```python
from build123d import *

# Parameters (mm, degrees)
F0_W     = 44.45
F0_H     = 38.1
F1_DEPTH = 19.05
F3_D     = 6.35
F3_DEPTH = 12.7
F3_TIP   = 1.9077324654
F5_D     = 6.35
F5_DEPTH = 12.7
F5_TIP   = 1.9077324654


with BuildPart() as f1:
    # F0 (on Right) → F1 (new body)
    with BuildSketch(Plane.YZ):
        with Locations((22.225, 19.05)):
            Rectangle(F0_W, F0_H)
    extrude(amount=F1_DEPTH)

    # F3
    with Locations(Plane.XY.offset(38.1)):
        with Locations((9.525, 22.225)):
            Hole(F3_D / 2, depth=F3_DEPTH)
            with Locations((0, 0, -(F3_DEPTH + F3_TIP / 2))):  # 118° drill point
                Cone(0, F3_D / 2, F3_TIP, mode=Mode.SUBTRACT)

    # F5
    with Locations(Plane(origin=(0, 0, 0), x_dir=(1, 0, 0), z_dir=(0, 0, -1))):
        with Locations((9.525, -12.7), (9.525, -31.75)):
            Hole(F5_D / 2, depth=F5_DEPTH)
            with Locations((0, 0, -(F5_DEPTH + F5_TIP / 2))):  # 118° drill point
                Cone(0, F5_D / 2, F5_TIP, mode=Mode.SUBTRACT)


solid = f1.part
```
Source: CAD feature listing. Evaluate the final solid. Frame: model axes, mm. A direction names the side the tool comes from. Give positions to 0.01 mm unless a question says otherwise; leave off trailing zeros. Loops run counter-clockwise (first coordinate to the right, second up) from the corner with the lowest first, then second, coordinate; pieces in that order, holes last. Notation, with made-up numbers: (-18, -36.75) - (14, -36.75) arc R20 ccw to (14, -11.75) - close; hole circle Ø2 at (-10.5, 71). An arc over 180 degrees is marked (long way). Use CSV: the item, a comma, the result in double quotes. Start each with the question number.
1. Ray query, L1, parallel to X at y = 12.7, z = 10; L2, parallel to Y at x = 7.75, z = 11.5; L3, parallel to X at y = 12, z = 7. Return the intervals inside material, ascending.
2. Section B-B (z = 29.5). Output: boundary loops of the cut face in (x, y) (3 decimals), then the cut area to 3 significant figures.
3. Section A-A (z = 3.5). Output: boundary loops of the cut face in (x, y) (3 decimals).
4. Reachability of faces 5 (the cylindrical face through (10.21, 34.85, 6.44)), 6 (the flat face through (0, 22, 19)), 7 (the cylindrical face through (9.938, 25.373, 31.661)) from +Z, -Z, +X, -X, +Y, -Y: full face, straight path, thin tool, end or side. Return the list, or none.
5. Pin query (flat end, axial travel): pin 1 (2 mm diameter, centred on x = 8.5, y = 22, fed in from +Z); pin 2 (5.5 mm diameter, centred on x = 9.525, y = 22.225, fed in from +Z). Return the tip coordinate at first contact, or that it passes through.
6. Draft query along Y for faces 1 (the flat face through (9, 22, 0)), 2 (the flat face through (9, 44.45, 19)), 3 (the flat face through (9, 0, 19)), 4 (the conical face through (9.453, 22.772, 23.824)). Return one class per face: +Y half, -Y half, draft (parallel to the pull), parting line (faces both ways), or undercut.
Response:
1,L1,"0 to 6.35, 12.7 to 19.05"
1,L2,"0 to 10.07, 15.33 to 29.12, 34.38 to 44.45"
1,L3,"0 to 6.43, 12.62 to 19.05"
2,outline,"(0, 0) - (19.05, 0) - (19.05, 44.45) - (0, 44.45) - close; hole circle Ø6.35 at (9.525, 22.225)"
2,area,"815 mm²"
3,outline,"(0, 0) - (19.05, 0) - (19.05, 44.45) - (0, 44.45) - close; hole circle Ø6.35 at (9.525, 12.7); hole circle Ø6.35 at (9.525, 31.75)"
4,face 5,"-Z"
4,face 6,"+Z, -Z, -X, +Y, -Y"
4,face 7,"+Z"
5,pin 1,"z = 24.72"
5,pin 2,"z = 25.14"
6,face 1,"draft"
6,face 2,"+Y half"
6,face 3,"-Y half"
6,face 4,"undercut"
